Source: CAD feature listing. Evaluate the final solid. Frame: model axes, mm. Give positions to 0.01 mm unless a question says otherwise; leave off trailing zeros. Order: outer loops, then holes, each group sorted by start corner. A loop starts at its lowest first (then second) coordinate and runs counter-clockwise, first axis right, second up. Notation, with made-up numbers: M 22.25,22.25 L 57.25,22.25 A28 cw 57.25,51.25 Z; hole C 30,6 d5. An arc over 180 degrees is marked long. Answer as a JSON object with one key per item and string values. Group by question number.
1. Section query A-A (x = -14.75). Output: boundary loops of the cut face in (y, z).
2. Material intervals for L1, parallel to Y at x = -14.25, z = 11.5; L2, parallel to X at y = -10, z = 48; L3, parallel to Y at x = -4.75, z = 84.5, sorted ascending. Write a range as [from, to].
3. Section query D-D (z = 19.5). Output: boundary loops of the cut face in (x, y).
4. Section query C-C (z = 123). Output: boundary loops of the cut face in (x, y).
5. Pin query (flat end, axial travel): P1, Ø1.8, axis at x = -6, z = 101, coming from the +Y side; P2, Ø6, axis at x = -16, z = 143.5, coming from the +Y side; P3, Ø5, axis at x = -14, y = -6.5, coming from the -Z side; P4, Ø4.5, axis at x = -12, y = 1, coming from the +Z side. Return the tip coordinate at first contact, or that it passes through.
6. Section query B-B (y = -6.75). Output: boundary loops of the cut face in (x, z).
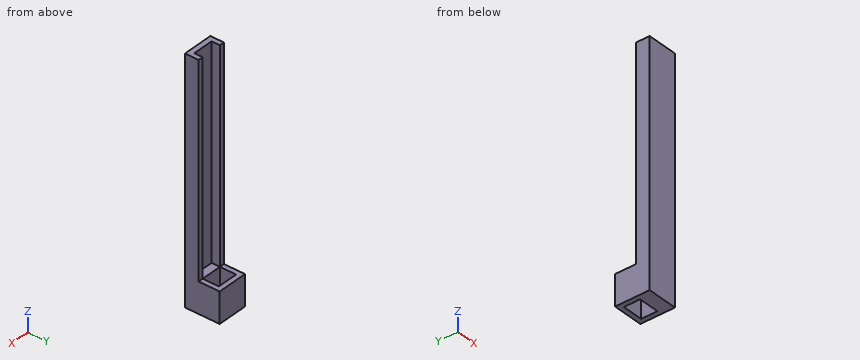
from build123d import *

# Parameters (mm, degrees)
SKETCH_2_W          = 22
SKETCH_2_H          = 25
SKETCH_2_W_2        = 15
SKETCH_2_H_2        = 11.7
EXTRUDE_1_DEPTH     = 22
SKETCH_3_W          = 22
SKETCH_3_H          = 9.8
EXTRUDE_2_DEPTH     = 150
SKETCH_4_W          = 15
SKETCH_4_H          = 150
CUT_EXTRUDE_1_DEPTH = 6


with BuildPart() as part:
    # 草圖2 → 填料-伸長1 (new body)
    with BuildSketch(Plane.XY):
        with Locations((-14.61342143, -7.059615385)):
            Rectangle(SKETCH_2_W, SKETCH_2_H)
        with Locations((-14.61342143, -3.909615385)):
            Rectangle(SKETCH_2_W_2, SKETCH_2_H_2, mode=Mode.SUBTRACT)
    extrude(amount=EXTRUDE_1_DEPTH)

    # 草圖3 → 填料-伸長2 (add)
    with BuildSketch(Plane.XY.offset(22)):
        with Locations((-14.61342143, -14.659615385)):
            Rectangle(SKETCH_3_W, SKETCH_3_H)
    extrude(amount=EXTRUDE_2_DEPTH)

    # 草圖4 → 除料-伸長1 (cut)
    with BuildSketch(Plane(origin=(0, -9.759615385, 0), x_dir=(1, 0, 0), z_dir=(0, 1, 0))):
        with Locations((-14.61342143, -97)):
            Rectangle(SKETCH_4_W, SKETCH_4_H)
    extrude(amount=-CUT_EXTRUDE_1_DEPTH, mode=Mode.SUBTRACT)


solid = part.part
Answer sheet:
{
 "1": {"outline": "M -19.56,0 L -9.76,0 L -9.76,22 L -15.76,22 L -15.76,172 L -19.56,172 Z; M 1.94,0 L 5.44,0 L 5.44,22 L 1.94,22 Z"},
 "2": {"L1": "[-19.56, -9.76], [1.94, 5.44]", "L2": "[-25.61, -22.11], [-7.11, -3.61]", "L3": "[-19.56, -9.76]"},
 "3": {"outline": "M -25.61,-19.56 L -3.61,-19.56 L -3.61,5.44 L -25.61,5.44 Z; hole M -22.11,-9.76 L -7.11,-9.76 L -7.11,1.94 L -22.11,1.94 Z"},
 "4": {"outline": "M -25.61,-19.56 L -3.61,-19.56 L -3.61,-9.76 L -7.11,-9.76 L -7.11,-15.76 L -22.11,-15.76 L -22.11,-9.76 L -25.61,-9.76 Z"},
 "5": {"P1": "y = -9.76", "P2": "y = -15.76", "P3": "through", "P4": "z = 22"},
 "6": {"outline": "M -25.61,0 L -22.11,0 L -22.11,22 L -25.61,22 Z; M -7.11,0 L -3.61,0 L -3.61,22 L -7.11,22 Z"}
}
